Model file for the job. Use its own axes, mm. A direction names the side the tool comes from. Coordinates: 2 decimals unless noted, no trailing zeros. Order: outer loops, then holes, each group sorted by start corner. A loop starts at its lowest first (then second) coordinate and runs counter-clockwise, first axis right, second up. Notation, with made-up numbers: (38, 14.25) -> (93, 14.25) arc R7 cw to (93, 27.25) -> close; hole circle Ø4 at (7, 35). An arc over 180 degrees is marked (long way). Write item = value, one per line. Start each with the question number.
Q1. Cut at B-B, the plane x = -22. List the corners of the cut face in (y, z).
Q2. Flat gauge pins, fed straight in: pin 1 (4.5 mm diameter, centred on x = -34, z = -18.5, fed in from +Y); pin 2 (2 mm diameter, centred on x = -20.5, z = -18.5, fed in from +Y); pin 3 (1.3 mm diameter, centred on x = -9, z = -17.5, fed in from +Y). Where does each tip first touch, or does it go through?
Q3. Mould opens along Y. For faces 1 (the face through (-18.446, -96, -18)), 2 (the face through (-22, -199, -10)), 3 (the face through (-21, -119, -16)), 4 (the face through (-15.946, -147, -18)) say: +Y half, -Y half, draft (parallel to the pull), parting line (faces both ways), or undercut.
Q4. 3-axis set-ups, long thin cutter, end or side, ignore diameter. For faces 5 (the face through (18.5, -130, -10)), 6 (the face through (-38.665, -178, -18)), 7 (the face through (-5.833, -97, -18)): which of +Z, -Z, +X, -X, +Y, -Y reach the whole face in a straight line?
Q5. Wall check: line 1 (X direction, y = -85, z = -18.5) (3 decimals); line 2 (Y direction, x = -20, z = -19); line 3 (Z direction, x = -31, y = -123). Give the ranges that are in metal, low to high. Write a range as from..to.
Q6. Cut at A-A, the plane y = -153.5. List the corners of the cut face in (x, z) (3 decimals).
Q7. Cut at D-D, the plane x = -9.5. List the corners of the cut face in (y, z).
Q8. Cut at C-C, the plane y = -113.5. List the corners of the cut face in (x, z) (3 decimals).
from build123d import *

# Parameters (mm, degrees)
SKETCH1_W           = 79
SKETCH1_H           = 140
BOSS_EXTRUDE1_DEPTH = 20
SKETCH3_W           = 5
SKETCH3_H           = 5
CUT_EXTRUDE1_DEPTH  = 131
SKETCH4_W           = 11
SKETCH4_H           = 25
CUT_EXTRUDE2_DEPTH  = 4
FILLET1_R           = 2
CHAMFER1_SIZE       = 0.5
SKETCH6_W           = 5.105326573
SKETCH6_H           = 5
CUT_EXTRUDE3_DEPTH  = 100
SKETCH7_W           = 10.105326573
SKETCH7_H           = 25
CUT_EXTRUDE4_DEPTH  = 4
FILLET2_R           = 2
CHAMFER2_SIZE       = 0.5
SKETCH8_W           = 6
SKETCH8_H           = 6
CUT_EXTRUDE5_DEPTH  = 103
SKETCH9_W           = 11
SKETCH9_H           = 25
CUT_EXTRUDE6_DEPTH  = 4.5
FILLET3_R           = 2
CHAMFER3_SIZE       = 2


with BuildPart() as part:
    # Sketch1 → Boss-Extrude1 (new body)
    with BuildSketch(Plane.XY):
        with Locations((-21, -129)):
            Rectangle(SKETCH1_W, SKETCH1_H)
    extrude(amount=-BOSS_EXTRUDE1_DEPTH)

    # Sketch3 → Cut-Extrude1 (cut)
    with BuildSketch(Plane(origin=(0, -59, 0), x_dir=(1, 0, 0), z_dir=(0, 1, 0))):
        with Locations((-33.165, 18.5)):
            Rectangle(SKETCH3_W, SKETCH3_H)
    extrude(amount=-CUT_EXTRUDE1_DEPTH, mode=Mode.SUBTRACT)

    # Sketch4 → Cut-Extrude2 (cut)
    with BuildSketch(Plane(origin=(0, 0, -20), x_dir=(-1, 0, 0), z_dir=(0, 0, -1))):
        with Locations((33.165, -177.5)):
            Rectangle(SKETCH4_W, SKETCH4_H)
    extrude(amount=-CUT_EXTRUDE2_DEPTH, mode=Mode.SUBTRACT)

    # Fillet1
    fillet1_edges = [part.edges().sort_by_distance(p)[0] for p in [
        (-38.665, -190, -18),
        (-27.665, -165, -18),
        (-38.665, -165, -18),
        (-27.665, -190, -18),
    ]]
    fillet(fillet1_edges, radius=FILLET1_R)

    # Chamfer1
    chamfer1_edges = [part.edges().sort_by_distance(p)[0] for p in [
        (-30.665, -165, -18),
        (-35.665, -165, -18),
    ]]
    chamfer(chamfer1_edges, length=CHAMFER1_SIZE)

    # Sketch6 → Cut-Extrude3 (cut)
    with BuildSketch(Plane(origin=(0, -59, 0), x_dir=(1, 0, 0), z_dir=(0, 1, 0))):
        with Locations((-20.998333333, 18.5)):
            Rectangle(SKETCH6_W, SKETCH6_H)
    extrude(amount=-CUT_EXTRUDE3_DEPTH, mode=Mode.SUBTRACT)

    # Sketch7 → Cut-Extrude4 (cut)
    with BuildSketch(Plane(origin=(0, 0, -20), x_dir=(-1, 0, 0), z_dir=(0, 0, -1))):
        with Locations((20.998333333, -146.5)):
            Rectangle(SKETCH7_W, SKETCH7_H)
    extrude(amount=-CUT_EXTRUDE4_DEPTH, mode=Mode.SUBTRACT)

    # Fillet2
    fillet2_edges = [part.edges().sort_by_distance(p)[0] for p in [
        (-26.05099662, -159, -18),
        (-15.945670047, -134, -18),
        (-26.05099662, -134, -18),
        (-15.945670047, -159, -18),
    ]]
    fillet(fillet2_edges, radius=FILLET2_R)

    # Chamfer2
    chamfer2_edges = [part.edges().sort_by_distance(p)[0] for p in [
        (-23.55099662, -134, -18),
        (-18.445670047, -134, -18),
    ]]
    chamfer(chamfer2_edges, length=CHAMFER2_SIZE - 0.0001)  # a hair under: the kernel refuses the full size

    # Sketch8 → Cut-Extrude5 (cut)
    with BuildSketch(Plane(origin=(0, -59, 0), x_dir=(1, 0, 0), z_dir=(0, 1, 0))):
        with Locations((-8.833333333, 18.5)):
            Rectangle(SKETCH8_W, SKETCH8_H)
    extrude(amount=-CUT_EXTRUDE5_DEPTH, mode=Mode.SUBTRACT)

    # Sketch9 → Cut-Extrude6 (cut)
    with BuildSketch(Plane(origin=(0, 0, -20), x_dir=(-1, 0, 0), z_dir=(0, 0, -1))):
        with Locations((8.833333333, -149.5)):
            Rectangle(SKETCH9_W, SKETCH9_H)
    extrude(amount=-CUT_EXTRUDE6_DEPTH, mode=Mode.SUBTRACT)

    # Fillet3
    fillet3_edges = [part.edges().sort_by_distance(p)[0] for p in [
        (-14.333333333, -162, -17.75),
        (-3.333333333, -137, -17.75),
        (-14.333333333, -137, -17.75),
        (-3.333333333, -162, -17.75),
    ]]
    fillet(fillet3_edges, radius=FILLET3_R)

    # Chamfer3
    chamfer3_edges = [part.edges().sort_by_distance(p)[0] for p in [
        (-60.5, -59, -10),
        (18.5, -59, -10),
        (18.5, -199, -10),
        (-60.5, -199, -10),
    ]]
    chamfer(chamfer3_edges, length=CHAMFER3_SIZE)


solid = part.part
Here are the results:
q1.outline = (-199, -20) -> (-159, -20) -> (-159, -16) -> (-59, -16) -> (-59, 0) -> (-199, 0) -> close
q2.pin_1 = -59
q2.pin_2 = -159
q2.pin_3 = -162
q3.face_1 = draft
q3.face_2 = -Y half
q3.face_3 = undercut
q3.face_4 = undercut
q4.face_5 = +Z, -Z, +X, +Y, -Y
q4.face_6 = -Z
q4.face_7 = -Z, +Y
q5.line_1 = -60.5..-35.665, -30.665..-23.551, -18.446..-11.833, -5.833..18.5
q5.line_2 = -199..-159
q5.line_3 = -16..0
q6.outline = (-60.5, -20) -> (-35.665, -20) -> (-35.665, -16) -> (-30.665, -16) -> (-30.665, -20) -> (-26.051, -20) -> (-26.051, -16) -> (-15.946, -16) -> (-15.946, -20) -> (-14.333, -20) -> (-14.333, -15.5) -> (-3.333, -15.5) -> (-3.333, -20) -> (18.5, -20) -> (18.5, 0) -> (-60.5, 0) -> close
q7.outline = (-199, -20) -> (-162, -20) -> (-162, -15.5) -> (-59, -15.5) -> (-59, 0) -> (-199, 0) -> close
q8.outline = (-60.5, -20) -> (-35.665, -20) -> (-35.665, -16) -> (-30.665, -16) -> (-30.665, -20) -> (-23.551, -20) -> (-23.551, -16) -> (-18.446, -16) -> (-18.446, -20) -> (-11.833, -20) -> (-11.833, -15.5) -> (-5.833, -15.5) -> (-5.833, -20) -> (18.5, -20) -> (18.5, 0) -> (-60.5, 0) -> close
